```python
from build123d import *

# Parameters (mm, degrees)
SKETCH1_R               = 3.175
BOSS_EXTRUDE1_DEPTH     = 25.4
SKETCH2_R               = 1.905
CUT_EXTRUDE1_DEPTH      = 12.7
CUT_EXTRUDE2_DEPTH      = 26.793821935
CUT_EXTRUDE2_DEPTH_BACK = 26.793821935
SKETCH3_R               = 1.905


with BuildPart() as part:
    # Sketch1 → Boss-Extrude1 (new body)
    with BuildSketch(Plane.XY):
        Circle(SKETCH1_R)
    extrude(amount=BOSS_EXTRUDE1_DEPTH)

    # Sketch2 → Cut-Extrude1 (cut)
    with BuildSketch(Plane.XY.offset(25.4)):
        Circle(SKETCH2_R)
    extrude(amount=-CUT_EXTRUDE1_DEPTH, mode=Mode.SUBTRACT)

    # Sketch3 → Cut-Extrude2 (cut, two sides: drawn at the far end of the back side and taken through both)
    with BuildSketch(Plane(origin=(0, 0, 0), x_dir=(0, 0, -1), z_dir=(1, 0, 0)).offset(-CUT_EXTRUDE2_DEPTH_BACK)):
        with Locations((-2.54, 0)):
            Circle(SKETCH3_R)
    extrude(amount=CUT_EXTRUDE2_DEPTH + CUT_EXTRUDE2_DEPTH_BACK, mode=Mode.SUBTRACT)


solid = part.part
```
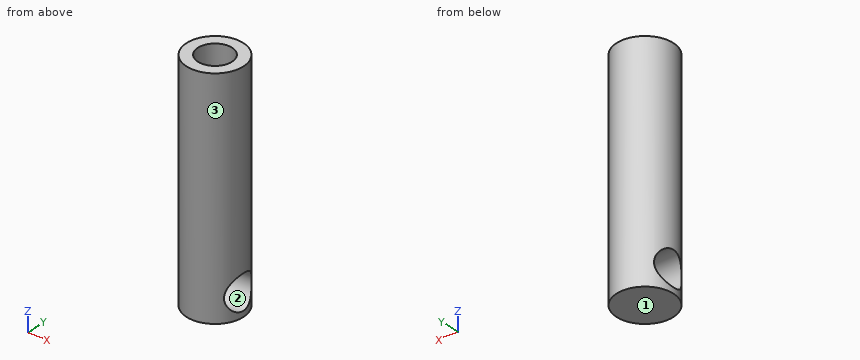
Check sheet for the modelled part. Datum: model origin and axes. Units: mm. Face numbers are marked on the shaded views. Give positions to 0.01 mm unless a question says otherwise; leave off trailing zeros. Order: outer loops, then holes, each group sorted by start corner. A loop starts at its lowest first (then second) coordinate and runs counter-clockwise, first axis right, second up. Notation, with made-up numbers: M -14.5,-17 L -10.5,-17 A11 cw -10.5,-12 Z; hole C -3,89.5 d8. An arc over 180 degrees is marked long. Answer in a Markdown table with one row per item.
1) Gauge pin test, flat ends, axial feed: P1, Ø1.5, axis at y = -0.5, z = 9.5, coming from the -X side (3 decimals); P2, Ø2, axis at x = -0.5, y = 0.5, coming from the +Z side; P3, Ø1.5, axis at y = 1.5, z = 3, coming from the +X side. Record the tip position at first contact, or that the pin passes through.
Filled sheet:
| item | result |
|---|---|
| P1 | stops at x = -3.175 |
| P2 | stops at z = 12.7 |
| P3 | stops at x = 2.81 |
2) Cross-section at D-D, the plane x = -1. Enter the section's corners in (y, z) (3 decimals), plus the area to 3 significant figures.
Filled sheet:
| item | result |
|---|---|
| outline | M -3.013,0 L 3.013,0 L 3.013,25.4 L 1.621,25.4 L 1.621,12.7 L -1.621,12.7 L -1.621,25.4 L -3.013,25.4 Z; hole C 0,2.54 d3.81 |
| area | 100 mm2 |
3) Thickness scan on L1, parallel to Z at x = 2, y = 0 (3 decimals); L2, parallel to Z at x = 1, y = 0 (3 decimals); L3, parallel to Y at x = 0, z = 20 (3 decimals). Record the ranges inside material, lowest first. Write a range as [from, to].
Filled sheet:
| item | result |
|---|---|
| L1 | z = [0, 0.635], [4.445, 25.4] |
| L2 | z = [0, 0.635], [4.445, 12.7] |
| L3 | y = [-3.175, -1.905], [1.905, 3.175] |
4) Release check for a two-part mould opening along Y. For the marked faces 1, 2 and 3 record: +Y half, -Y half, draft (parallel to the pull), parting line (faces both ways), or undercut.
Filled sheet:
| item | result |
|---|---|
| face 1 | draft |
| face 2 | undercut |
| face 3 | parting line |
5) Cross-section at B-B, the plane x = 0. Enter the section's corners in (y, z) (3 decimals), plus the area to 3 significant figures.
Filled sheet:
| item | result |
|---|---|
| outline | M -3.175,0 L 3.175,0 L 3.175,25.4 L 1.905,25.4 L 1.905,12.7 L -1.905,12.7 L -1.905,25.4 L -3.175,25.4 Z; hole C 0,2.54 d3.81 |
| area | 102 mm2 |
6) Cross-section at C-C, the plane z = 2.54. Enter the section's corners in (x, y) (3 decimals), plus the area to 3 significant figures.
Filled sheet:
| item | result |
|---|---|
| outline | M -2.54,-1.905 A3.175 ccw 2.54,-1.905 Z; M -2.54,1.905 L 2.54,1.905 A3.175 ccw Z |
| area | 9.02 mm2 |
7) Cross-section at A-A, the plane y = 0. Enter the section's corners in (x, z) (3 decimals), plus the area to 3 significant figures.
Filled sheet:
| item | result |
|---|---|
| outline | M -3.175,0 L 3.175,0 L 3.175,0.635 L -3.175,0.635 Z; M -3.175,4.445 L 3.175,4.445 L 3.175,25.4 L 1.905,25.4 L 1.905,12.7 L -1.905,12.7 L -1.905,25.4 L -3.175,25.4 Z |
| area | 88.7 mm2 |
